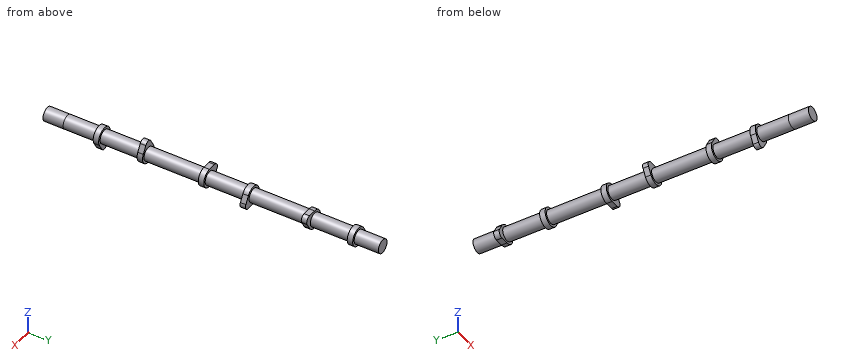
from build123d import *
from build123d.topology import SkipClean

# Parameters (mm, degrees)
BOSS_EXTRUDE1_DEPTH   = 3.81
BODY_MOVE_COPY2_ANGLE = 180
BOSS_EXTRUDE2_START   = 25.4
SKETCH2_R             = 9.5
BOSS_EXTRUDE2_DEPTH   = 73.025
LPATTERN1_COUNT       = 3
LPATTERN1_PITCH       = 146.05
BODY_MOVE_COPY3_ANGLE = 120
BODY_MOVE_COPY4_ANGLE = 120
SKETCH3_R             = 9.5
BOSS_EXTRUDE3_DEPTH   = 27.94
SCALE1_SCALE          = 0.51948


with BuildPart() as part:
    # Sketch1 → Boss-Extrude1 (new, symmetric)
    with BuildSketch(Plane(origin=(0, 0, 0), x_dir=(1, 0, 0), z_dir=(0, 1, 0))):
        with BuildLine():
            Line((-5.499261314, 15.875), (-10.998522628, 6.35))
            ThreePointArc((-10.998522628, 6.35), (0, -12.7), (10.998522628, 6.35))
            Line((10.998522628, 6.35), (5.499261314, 15.875))
            ThreePointArc((5.499261314, 15.875), (0, 19.05), (-5.499261314, 15.875))
        make_face()
    extrude(amount=BOSS_EXTRUDE1_DEPTH, both=True)


with BuildPart() as body_2:
    # Body-Move_Copy1: copy of part
    add(part.part.moved(Location((0, 60.96, 0))))


with BuildPart() as body_2_1:
    # Body-Move_Copy2: moved
    add(body_2.part.rotate(Axis((0, 0, 0), (0, 1, 0)), BODY_MOVE_COPY2_ANGLE))


with BuildPart() as part_1:
    add(part.part)

    add(body_2_1.part)  # Boss-Extrude2 merges body 2
    # Sketch2 → Boss-Extrude2 (add, symmetric)
    with BuildSketch(Plane(origin=(0, 0, 0), x_dir=(1, 0, 0), z_dir=(0, 1, 0)).offset(BOSS_EXTRUDE2_START)):
        with Locations(Location((0, 0, 0), (0, 0, 270))):
            Circle(SKETCH2_R)
    extrude(amount=BOSS_EXTRUDE2_DEPTH, both=True)


with BuildPart() as lpattern1_1:
    # LPattern1: pattern copy
    add(part_1.part.moved(Location(Vector(0, 1, 0) * (1 * LPATTERN1_PITCH))))


with BuildPart() as lpattern1_2:
    # LPattern1: pattern copy
    add(part_1.part.moved(Location(Vector(0, 1, 0) * (2 * LPATTERN1_PITCH))))


with BuildPart() as lpattern1_1_1:
    # Body-Move_Copy3: moved
    add(lpattern1_1.part.rotate(Axis((0, 0, 0), (0, 1, 0)), BODY_MOVE_COPY3_ANGLE))


with BuildPart() as lpattern1_2_1:
    # Body-Move_Copy4: moved
    add(lpattern1_2.part.rotate(Axis((0, 0, 0), (0, -1, 0)), BODY_MOVE_COPY4_ANGLE))


with BuildPart() as part_2:
    with SkipClean():  # the faces are left unmerged after this step: merging them gives an invalid solid
        add(part_1.part)

        # Sketch3 → Boss-Extrude3 (add)
        with BuildSketch(Plane.XZ.offset(47.625)):
            with Locations(Location((0, 0, 0), (0, 0, 210))):
                Circle(SKETCH3_R)
        extrude(amount=BOSS_EXTRUDE3_DEPTH)

    # Combine1: union LPattern1_1, LPattern1_2
    add(lpattern1_1_1.part)
    add(lpattern1_2_1.part)


with BuildPart() as part_3:
    # Scale1: scaled about (0, 159.303825553, 0)
    add(part_2.part.scale(SCALE1_SCALE).moved(Location((0, 76.548674255, 0))))


solid = part_3.part
Geometry check sheet. Reference: the model listing, model coordinates, mm. Round coordinates to 2 decimals unless told otherwise and drop trailing zeros. Write each loop counter-clockwise with the first axis right and the second up, starting at its lowest first coordinate (ties: lowest second). Pieces come first, ordered by that corner, then holes. Notation, with made-up numbers: (23.5, 24) -> (80.5, 24) arc R19 ccw to (80.5, 38) -> close; hole circle Ø3 at (-24, 28.5). An arc over 180 degrees is marked (long way). One line per item, written item: value. Start each with the question number.
(1) Cross-section at A-A, the plane y = 147.5. Record the cut outline in (x, z).
(2) Scan lines: line 1 (Y direction, x = -2, z = 4.75); line 2 (Y direction, x = 3.25, z = 6); line 3 (Y direction, x = 3.25, z = -7). Record each from-to range of solid material in increasing order. Write a range as [from, to].
(3) Go/stop test with flat-tipped pins: pin 1 Ø2 at (x, y) = (1.5, 227.5) entering from +Z; pin 2 Ø4.5 at (x, y) = (2, 185) entering from -Z; pin 3 Ø2 at (y, z) = (203.5, -2) entering from +X. Record where each tip stops, or that it passes through.
Answer:
1. outline: circle Ø9.87 at (0, 0)
2. line 1: [74.57, 78.53], [106.24, 110.2], [150.44, 154.4], [182.11, 186.07], [226.31, 230.27], [257.98, 261.94]
2. line 2: [106.24, 110.2], [226.31, 230.27]
2. line 3: [74.57, 78.53]
3. pin 1: z = 6.6
3. pin 2: z = -6.6
3. pin 3: x = 4.83
